The model under review builds one solid part; all positions refer to its coordinate system, in mm. Coordinates: 2 decimals unless noted, no trailing zeros. Order: outer loops, then holes, each group sorted by start corner. A loop starts at its lowest first (then second) coordinate and runs counter-clockwise, first axis right, second up. Notation, with made-up numbers: (8, -28) -> (46, -28) arc R24 cw to (46, -9) -> close; hole circle Ø10 at (-14.75, 39). An arc over 180 degrees is marked (long way). Use one line per item in the form item = value. Start each with the question number.
(1) Take a section at C-C (y = -2). State the section outline as (x, z) points.
(2) Insertion check: pin 1 Ø1.6 at (x, z) = (-52, 2) entering from +Y; pin 2 Ø1.6 at (y, z) = (-3.5, 2.5) entering from -X; pin 3 Ø1 at (y, z) = (-2.5, 1.5) entering from +X. Each pin has a flat end and moves straight along its axis. Give the tip position at first contact, or say it passes through.
(3) Take a section at A-A (z = 0.55). State the section outline as (x, y) points, then the cut area to 3 significant figures.
(4) Take a section at D-D (x = 15.5). State the section outline as (y, z) points, then the cut area to 3 significant figures.
(5) Take a section at B-B (x = -4.5). State the section outline as (y, z) points, then the cut area to 3 significant figures.
(6) Wall thickness on line 1 along Y through (x, z) = (-5, 1.45); line 2 along X through (y, z) = (4, 1); line 3 along Y through (x, z) = (15, 2.1): over which ranges is each line inside the solid? List them lowest first.
Autodesk Inventor part; units mm, degrees
ref_plane "YZ Plane" through (0, 0, 0) normal (1, 0, 0) x (0, 1, 0)
ref_plane "XZ Plane" through (0, 0, 0) normal (0, 1, 0) x (-1, 0, 0)
ref_plane "XY Plane" through (0, 0, 0) normal (0, 0, 1) x (1, 0, 0)
sketch "Boceto1" plane through (0, 0, 0) normal (0, 0, 1) x (1, 0, 0)
  line L0 (-53.18, -36.59) -> (53.18, -36.59)
  line L1 (53.18, -36.59) -> (53.18, 36.59)
  line L2 (53.18, 36.59) -> (-53.18, 36.59)
  line L3 (-53.18, 36.59) -> (-53.18, -36.59)
  line L4 (-53.18, -36.59) -> (53.18, 36.59) construction
  line L5 (53.18, -36.59) -> (-53.18, 36.59) construction
  line L6 (-19.9778, -36.59) -> (30.0222, -36.59)
  line L7 (-25, 39.77) -> (25, 39.77)
  line L8 (25, 39.77) -> (25, 36.59)
  line L9 (25, 36.59) -> (-25, 36.59)
  line L10 (-25, 36.59) -> (-25, 39.77)
  line L11 (-53.18, 16.59) -> (-50, 16.59)
  line L12 (-50, 16.59) -> (-50, -13.41)
  line L13 (-50, -13.41) -> (-53.18, -13.41)
  line L14 (-53.18, -13.41) -> (-53.18, 16.59)
  line L15 (50, 16.59) -> (53.18, 16.59)
  line L16 (53.18, 16.59) -> (53.18, -13.41)
  line L17 (53.18, -13.41) -> (50, -13.41)
  line L18 (50, -13.41) -> (50, 16.59)
  line L19 (-25, -33.41) -> (25, -33.41)
  line L20 (25, -33.41) -> (25, -36.59)
  line L21 (25, -36.59) -> (-25, -36.59)
  line L22 (-25, -36.59) -> (-25, -33.41)
  line L23 (-7.5, 5) -> (7.5, 5)
  line L24 (7.5, 5) -> (7.5, 8.18)
  line L25 (7.5, 8.18) -> (-7.5, 8.18)
  line L26 (-7.5, 8.18) -> (-7.5, 5)
  line L27 (-7.5, 5) -> (7.5, 8.18) construction
  line L28 (7.5, 5) -> (-7.5, 8.18) construction
  point P0 (0, 0)
  point P1 (0, 6.59)
  dimension "d0" = 106.36
  dimension "d3" = 73.18
  dimension "d4" = 3.18
  dimension "d5" = 50
  dimension "d6" = 25
  dimension "d8" = 30
  dimension "d9" = 30
  dimension "d10" = 3.18
  dimension "d11" = 20
  dimension "d12" = 20
  dimension "d13" = 50
  dimension "d14" = 25
  dimension "d17" = 15
  dimension "d18" = 3.18
  dimension "d19" = 40
  dimension "d20" = 7.5
extrude "Extrusión1" add sketch "Boceto1" along normal blind 3.18 contours L3 L13 L12 L11 L2 L1 L15 L18 L17 L0 L20 L19 L22 | L10 L7 L8 L2
properties part number "BASE_TAPAFIJA"
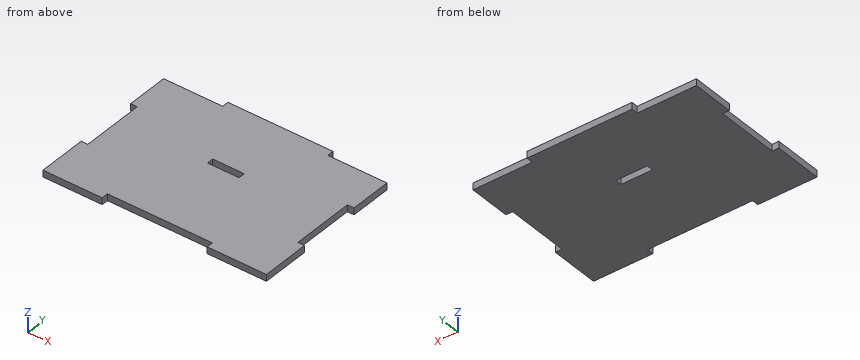
Findings:
q1.outline = (-50, 0) -> (50, 0) -> (50, 3.18) -> (-50, 3.18) -> close
q2.pin_1 = 36.59
q2.pin_2 = -50
q2.pin_3 = 50
q3.outline = (-53.18, -36.59) -> (-25, -36.59) -> (-25, -33.41) -> (25, -33.41) -> (25, -36.59) -> (53.18, -36.59) -> (53.18, -13.41) -> (50, -13.41) -> (50, 16.59) -> (53.18, 16.59) -> (53.18, 36.59) -> (25, 36.59) -> (25, 39.77) -> (-25, 39.77) -> (-25, 36.59) -> (-53.18, 36.59) -> (-53.18, 16.59) -> (-50, 16.59) -> (-50, -13.41) -> (-53.18, -13.41) -> close; hole (-7.5, 5) -> (7.5, 5) -> (7.5, 8.18) -> (-7.5, 8.18) -> close
q3.area = 7,540 mm²
q4.outline = (-33.41, 0) -> (39.77, 0) -> (39.77, 3.18) -> (-33.41, 3.18) -> close
q4.area = 233 mm²
q5.outline = (-33.41, 0) -> (5, 0) -> (5, 3.18) -> (-33.41, 3.18) -> close; (8.18, 0) -> (39.77, 0) -> (39.77, 3.18) -> (8.18, 3.18) -> close
q5.area = 223 mm²
q6.line_1 = -33.41 to 5, 8.18 to 39.77
q6.line_2 = -50 to 50
q6.line_3 = -33.41 to 39.77
